Can you work these out from the model? Positions are in its coordinate system, mm. A direction names the side the tool comes from. Give positions to 0.01 mm unless a question says otherwise; leave off trailing zeros. Answer as a JSON object with one key per item and string values.
```python
from build123d import *

# Parameters (mm, degrees)
EXTRUDE_1_DEPTH     = 10
SKETCH_2_W          = 6.5
SKETCH_2_H          = 6.5
CUT_EXTRUDE_1_DEPTH = 10


with BuildPart() as part:
    # 草图1 → 凸台-拉伸1 (new body)
    with BuildSketch(Plane.XY):
        with BuildLine():
            add(Edge.make_bspline(
                [(-19, 0), (-9.5, 33), (0, 33)],
                knots=[0, 0, 0, 0.5, 0.5, 0.5], degree=2))
            Line((-19, 0), (0, 0))
            Line((0, 0), (0, 33))
        make_face()
        with BuildLine():
            Line((0, 33), (0, 0))
            Line((0, 0), (19, 0))
            add(Edge.make_bspline(
                [(0, 33), (9.5, 33), (19, 0)],
                knots=[0.5, 0.5, 0.5, 1, 1, 1], degree=2))
        make_face()
    extrude(amount=EXTRUDE_1_DEPTH)

    # 草图2 → 切除-拉伸1 (cut)
    with BuildSketch(Plane(origin=(0, 0, 0), x_dir=(-1, 0, 0), z_dir=(0, 0, -1))):
        with Locations((-3.75, 18.75)):
            Rectangle(SKETCH_2_W, SKETCH_2_H)
        with Locations((-3.75, 11.25)):
            Rectangle(SKETCH_2_W, SKETCH_2_H)
        with Locations((3.75, 11.25)):
            Rectangle(SKETCH_2_W, SKETCH_2_H)
        with Locations((3.75, 18.75)):
            Rectangle(SKETCH_2_W, SKETCH_2_H)
    extrude(amount=-CUT_EXTRUDE_1_DEPTH, mode=Mode.SUBTRACT)


solid = part.part
```
1) For faces 4 (the flat face through (0, 14, 0)), 5 (the flat face through (-4, 8, 5)), which set-ups out of +Z, -Z, +X, -X, +Y, -Y let a thin tool reach every point of the face, with its end or its side?
Answer list:
{"face 4": "-Z, +X, -X, +Y, -Y", "face 5": "+Z, -Z"}
2) Suppose I cut it at A-A, the plane y = 10. Give the number of separate pieces and of enclosed holes in the cut face, and give its area (3 significant figures).
Answer list:
{"separate pieces": "3", "enclosed holes": "0", "area": "187 mm^2"}
3) If we mould it in two halves opening along Y, with no side actions, what happens to faces 1 (the flat face through (0, 14, 10)), 2 (the flat face through (0, 0, 5)), 3 (the flat face through (4, 22, 5))? For each: +Y half, -Y half, draft (parallel to the pull), parting line (faces both ways), or undercut.
Answer list:
{"face 1": "draft", "face 2": "-Y half", "face 3": "undercut"}
4) Please list where these lines run through material, in increasing order: line 1 along Y through (x, z) = (4.5, 3.75); line 2 along Y through (x, z) = (-3.5, 7.25); line 3 along X through (y, z) = (10, 7.25). Write a range as from..to.
Answer list:
{"line 1": "0..8, 14.5..15.5, 22..31.15", "line 2": "0..8, 14.5..15.5, 22..31.88", "line 3": "-15.86..-7, -0.5..0.5, 7..15.86"}
5) Will these pins go through, and if not, where does the flat tip stop? pin 1 Ø2 at (x, z) = (0.5, 7.5) entering from +Y; pin 2 Ø2 at (y, z) = (20.5, 3) entering from -X; pin 3 Ø3 at (y, z) = (19.5, 4) entering from +X; pin 4 Ø3 at (y, z) = (12, 7) entering from +X.
Answer list:
{"pin 1": "y = 33", "pin 2": "x = -12.15", "pin 3": "x = 12.81", "pin 4": "x = 15.69"}
